from build123d import *

# Parameters (mm, degrees)
F0_R      = 65.5
F1_DEPTH  = 13
F2_R      = 44.6
F2_R_2    = 34.6
F3_DEPTH  = 5
F4_R      = 34.6
F5_DEPTH  = 25
F7_DEPTH  = 8
F8_W      = 88.3397431672
F8_H      = 2
F9_DEPTH  = 2
F10_W     = 78
F10_H     = 2
F11_DEPTH = 2
F12_W     = 89.867619957
F12_H     = 2
F13_DEPTH = 2
F8_W_2    = 3.5278767898
F14_DEPTH = 2


with BuildPart() as f1:
    # F0 (on Top) → F1 (new body)
    with BuildSketch(Plane.XY):
        Circle(F0_R)
    extrude(amount=F1_DEPTH)

    # F2 (on Top) → F3 (cut)
    with BuildSketch(Plane.XY):
        Circle(F2_R)
        Circle(F2_R_2, mode=Mode.SUBTRACT)
        Circle(F2_R_2)
    extrude(amount=F3_DEPTH, mode=Mode.SUBTRACT)

    # F4 (on face) → F5 (cut)
    with BuildSketch(Plane(origin=(0, 0, 0), x_dir=(1, 0, 0), z_dir=(0, 0, -1))):
        Circle(F4_R)
    extrude(amount=-F5_DEPTH, mode=Mode.SUBTRACT)

    # F6 (on face) → F7 (cut)
    with BuildSketch(Plane.XY.offset(13)):
        with BuildLine():
            ThreePointArc((-34.6, 0), (0, 34.6), (34.6, 0))
            Line((34.6, 0), (40, 0))
            Line((40, 0), (40, 40))
            Line((40, 40), (-40, 40))
            Line((-40, 40), (-40, 0))
            Line((-40, 0), (-34.6, 0))
        make_face()
        with BuildLine():
            Line((40, 0), (34.6, 0))
            ThreePointArc((34.6, 0), (0, -34.6), (-34.6, 0))
            Line((-34.6, 0), (-40, 0))
            Line((-40, 0), (-40, -51.867619957))
            ThreePointArc((-40, -51.867619957), (0, -65.5), (40, -51.867619957))
            Line((40, -51.867619957), (40, 0))
        make_face()
    extrude(amount=-F7_DEPTH, mode=Mode.SUBTRACT)

    # F8 (on face) → F9 (join)
    with BuildSketch(Plane.YZ.offset(-40)):
        with Locations((-4.1698715836, 12)):
            Rectangle(F8_W, F8_H)
    extrude(amount=F9_DEPTH)

    # F10 (on face) → F11 (join)
    with BuildSketch(Plane.XZ.offset(-40)):
        with Locations((1, 12)):
            Rectangle(F10_W, F10_H)
    extrude(amount=F11_DEPTH)

    # F12 (on face) → F13 (join)
    with BuildSketch(Plane(origin=(40, 0, 0), x_dir=(0, -1, 0), z_dir=(-1, 0, 0))):
        with Locations((6.9338099785, 12)):
            Rectangle(F12_W, F12_H)
    extrude(amount=F13_DEPTH)

    # F8 (on face) → F14 (join)
    with BuildSketch(Plane.YZ.offset(-40)):
        with Locations((-4.1698715836, 12)):
            Rectangle(F8_W, F8_H)
        with Locations((-50.1036815621, 12)):
            Rectangle(F8_W_2, F8_H)
    extrude(amount=F14_DEPTH)


solid = f1.part
Input: part model. Units: mm. Frame: model coordinates. A direction names the side the tool comes from. Round coordinates to 2 decimals unless told otherwise and drop trailing zeros. Order: outer loops, then holes, each group sorted by start corner. A loop starts at its lowest first (then second) coordinate and runs counter-clockwise, first axis right, second up. Notation, with made-up numbers: (61.25, -29) - (101.25, -29) arc R36 ccw to (101.25, 7) - close; hole circle Ø11 at (-8.5, 16). An arc over 180 degrees is marked (long way). Answer as a JSON object with one key per item and string values. Group by question number.
(1) Pin query (flat end, axial travel): P1, Ø3, axis at x = 0.5, z = 2, coming from the +Y side; P2, Ø2.5, axis at x = 41.5, y = 9.5, coming from the -Z side; P3, Ø10, axis at x = -30.5, y = 30.5, coming from the +Z side; P4, Ø8, axis at x = -49, y = 2, coming from the -Z side. Return the tip coordinate at first contact, or that it passes through.
(2) Cut plane D-D (y = -31). Return loops of the section in (x, z).
(3) Draft query along X for faces 4 (the face through (-40, -5, 8)), 5 (the face through (14, -43, 0)), 6 (the face through (-8.527, 64.943, 6.409)). Return one class per face: released by +X, released by -X, zero draft, split by the parting line, or undercut.
(4) Reachability of faces 1 (the face through (1, 47, 13)), 2 (the face through (42.54, 13.4, 2.46)), 3 (the face through (-35, 35, 5)) from +Z, -Z, +X, -X, +Y, -Y: full face, straight path, thin tool, end or side. Return the list, or none.
(5) Material intervals for probe 1 along Y at (x, z) = (0, 1.2); probe 2 along X at (y, z) = (-33, 7.5), sorted ascending. Write a range as from..to.
(6) Cut plane C-C (z = 2.75). Return loops of the section in (x, y).
(7) Cut plane A-A (y = 0). Return loops of the section in (x, z).
(8) Cut plane B-B (x = 0). Return loops of the section in (y, z), then the cut area to 3 significant figures.
Here are the results:
{
 "1": {"P1": "stops at y = 65.5", "P2": "stops at z = 5", "P3": "stops at z = 5", "P4": "stops at z = 0"},
 "2": {"outline": "(-57.7, 0) - (-32.06, 0) - (-32.06, 5) - (-40, 5) - (-40, 11) - (-38, 11) - (-38, 13) - (-57.7, 13) - close; (32.06, 0) - (57.7, 0) - (57.7, 13) - (38, 13) - (38, 11) - (40, 11) - (40, 5) - (32.06, 5) - close"},
 "3": {"face 4": "undercut", "face 5": "zero draft", "face 6": "split by the parting line"},
 "4": {"face 1": "+Z, +X, -X, +Y, -Y", "face 2": "-Z", "face 3": "-Y"},
 "5": {"probe 1": "y = -65.5..-44.6, 44.6..65.5", "probe 2": "x = -56.58..-40, 40..56.58"},
 "6": {"outline": "circle Ø131 at (0, 0); hole circle Ø89.2 at (0, 0)"},
 "7": {"outline": "(-65.5, 0) - (-44.6, 0) - (-44.6, 5) - (-40, 5) - (-40, 11) - (-38, 11) - (-38, 13) - (-65.5, 13) - close; (38, 11) - (40, 11) - (40, 5) - (44.6, 5) - (44.6, 0) - (65.5, 0) - (65.5, 13) - (38, 13) - close"},
 "8": {"outline": "(-65.5, 0) - (-44.6, 0) - (-44.6, 5) - (-65.5, 5) - close; (38, 11) - (40, 11) - (40, 5) - (44.6, 5) - (44.6, 0) - (65.5, 0) - (65.5, 13) - (38, 13) - close", "area": "417 mm^2"}
}
